Verification items for the finished model (mm, model axes). A direction names the side the tool comes from. Give positions to 0.01 mm unless a question says otherwise; leave off trailing zeros. Order: outer loops, then holes, each group sorted by start corner. A loop starts at its lowest first (then second) coordinate and runs counter-clockwise, first axis right, second up. Notation, with made-up numbers: (63, -21.75) - (86, -21.75) arc R22 cw to (86, -2.75) - close; hole circle Ø9 at (-23, -6.75). An arc over 180 degrees is marked (long way). Answer as a JSON object with one key per item and string values.
```python
from build123d import *

# Parameters (mm, degrees)
SKETCH1_R           = 14
SKETCH1_R_2         = 2.75
BOSS_EXTRUDE1_DEPTH = 17
SKETCH2_R           = 2.65
CUT_EXTRUDE1_DEPTH  = 10
CHAMFER1_SIZE       = 1


with BuildPart() as part:
    # Sketch1 → Boss-Extrude1 (new, symmetric)
    with BuildSketch(Plane.XY):
        Polygon((15.46675804, -22), (-15.46675804, -22), (-35, 1.278811281), (-35, 30), (35, 30), (35, 1.278811281), align=None)
        Circle(SKETCH1_R, mode=Mode.SUBTRACT)
        with Locations((-13.435028843, -13.435028843)):
            Circle(SKETCH1_R_2, mode=Mode.SUBTRACT)
        with Locations((-19, 0)):
            Circle(SKETCH1_R_2, mode=Mode.SUBTRACT)
        with Locations(Location((-13.435028843, 13.435028843, 0), (0, 0, 180))):
            Circle(SKETCH1_R_2, mode=Mode.SUBTRACT)
        with Locations((13.435028843, 13.435028843)):
            Circle(SKETCH1_R_2, mode=Mode.SUBTRACT)
        with Locations(Location((19, 0, 0), (0, 0, 180))):
            Circle(SKETCH1_R_2, mode=Mode.SUBTRACT)
        with Locations(Location((13.435028843, -13.435028843, 0), (0, 0, 180))):
            Circle(SKETCH1_R_2, mode=Mode.SUBTRACT)
    extrude(amount=BOSS_EXTRUDE1_DEPTH, both=True)

    # Sketch2 → Cut-Extrude1 (cut)
    with BuildSketch(Plane(origin=(0, 30, 0), x_dir=(1, 0, 0), z_dir=(0, 1, 0))):
        with Locations(Location((-29, 11, 0), (0, 0, 180))):
            Circle(SKETCH2_R)
        with Locations(Location((-29, -11, 0), (0, 0, 180))):
            Circle(SKETCH2_R)
        with Locations(Location((29, -11, 0), (0, 0, 180))):
            Circle(SKETCH2_R)
        with Locations(Location((29, 11, 0), (0, 0, 180))):
            Circle(SKETCH2_R)
    extrude(amount=-CUT_EXTRUDE1_DEPTH, mode=Mode.SUBTRACT)

    # Chamfer1
    chamfer1_edges = [part.edges().sort_by_distance(p)[0] for p in [
        (-35, 15.639405641, 17),
        (-25.23337902, -10.360594359, 17),
        (25.23337902, -10.360594359, 17),
        (35, 15.639405641, 17),
        (25.23337902, -10.360594359, -17),
        (-25.23337902, -10.360594359, -17),
        (-35, 15.639405641, -17),
        (35, 15.639405641, -17),
    ]]
    chamfer(chamfer1_edges, length=CHAMFER1_SIZE)


solid = part.part
```
(1) Section check D-D (z = 11). Record the cut outline in (x, y), then the cut area to 3 significant figures.
Computed values:
{"outline": "(-35, 1.28) - (-15.47, -22) - (15.47, -22) - (35, 1.28) - (35, 30) - (31.65, 30) - (31.65, 20) - (26.35, 20) - (26.35, 30) - (-26.35, 30) - (-26.35, 20) - (-31.65, 20) - (-31.65, 30) - (-35, 30) - close; hole circle Ø5.5 at (-19, 0); hole circle Ø5.5 at (-13.44, -13.44); hole circle Ø5.5 at (-13.44, 13.44); hole circle Ø28 at (0, 0); hole circle Ø5.5 at (13.44, -13.44); hole circle Ø5.5 at (13.44, 13.44); hole circle Ø5.5 at (19, 0)", "area": "2,320 mm²"}
(2) Gauge pin test, flat ends, axial feed: pin 1 Ø6 at (x, z) = (-21, 6.5) entering from -Y; pin 2 Ø10 at (y, z) = (-14.5, 10.5) entering from -X; pin 3 Ø3 at (x, z) = (29, 11) entering from +Y. Record the tip position at first contact, or that the pin passes through.
Computed values:
{"pin 1": "stops at y = -18.98", "pin 2": "stops at x = -25.96", "pin 3": "stops at y = 20"}
(3) Access from +Z, -Z, +X, -X, +Y, -Y to the whole of each face (thin tool, end or side, straight path). Record for faces 1 (the cylindrical face through (-26.353, 25.07, 11.117)), 2 (the flat face through (0, 16, 17)).
Computed values:
{"face 1": "+Y", "face 2": "+Z, +X, -X, +Y, -Y"}
(4) Section check B-B (x = 0). Record the cut outline in (y, z), then the cut area to 3 significant figures.
Computed values:
{"outline": "(-22, -17) - (-14, -17) - (-14, 17) - (-22, 17) - close; (14, -17) - (30, -17) - (30, 17) - (14, 17) - close", "area": "816 mm²"}
(5) Section check C-C (y = 7.5). Record the cut outline in (x, z).
Computed values:
{"outline": "(-35, -16) - (-34, -17) - (-11.82, -17) - (-11.82, 17) - (-34, 17) - (-35, 16) - close; (11.82, -17) - (34, -17) - (35, -16) - (35, 16) - (34, 17) - (11.82, 17) - close"}
(6) Section check A-A (y = 27). Record the cut outline in (x, z), then the cut area to 3 significant figures.
Computed values:
{"outline": "(-35, -16) - (-34, -17) - (34, -17) - (35, -16) - (35, 16) - (34, 17) - (-34, 17) - (-35, 16) - close; hole circle Ø5.3 at (-29, -11); hole circle Ø5.3 at (-29, 11); hole circle Ø5.3 at (29, -11); hole circle Ø5.3 at (29, 11)", "area": "2,290 mm²"}
(7) Release check for a two-part mould opening along Z. For faces 3 (the flat face through (0, 16, -17)), 4 (the cylindrical face through (11.408, 15.294, -0.238)), 5 (the cylindrical face through (31.647, 25.07, -10.883)) record: pulls with the +Z half, pulls with the -Z half, needs draft (parallel to the pull), parting line crosses it, or undercut.
Computed values:
{"face 3": "pulls with the -Z half", "face 4": "needs draft", "face 5": "undercut"}
(8) Material ranges on line 1 along X through (y, z) = (-11, 0); line 2 along Y through (x, z) = (-15, -11); line 3 along X through (y, z) = (26, -13), recorded low to high. Write a range as [from, to].
Computed values:
{"line 1": "x = [-24.7, -14.71], [-12.16, -8.66], [8.66, 12.16], [14.71, 24.7]", "line 2": "y = [-22, -15.7], [-11.17, 11.17], [15.7, 30]", "line 3": "x = [-35, -30.74], [-27.26, 27.26], [30.74, 35]"}
